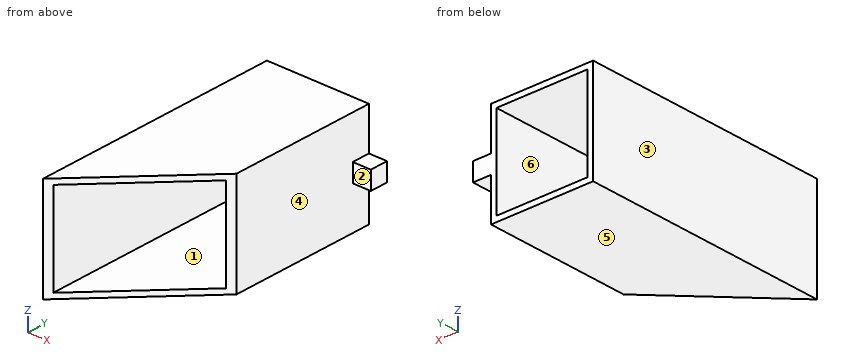
from build123d import *

# Parameters (mm, degrees)
CROQUIS1_W              = 56.5
CROQUIS1_H              = 56.5
SALIENTE_EXTRUIR1_DEPTH = 81.9
SALIENTE_EXTRUIR2_DEPTH = 56.5
VACIADO4_T              = -3
CROQUIS3_W              = 10
CROQUIS3_H              = 10
SALIENTE_EXTRUIR3_DEPTH = 10


with BuildPart() as part:
    # Croquis1 → Saliente-Extruir1 (new body)
    with BuildSketch(Plane(origin=(0, 0, 0), x_dir=(1, 0, 0), z_dir=(0, 1, 0))):
        with Locations((28.25, 28.25)):
            Rectangle(CROQUIS1_W, CROQUIS1_H)
    extrude(amount=SALIENTE_EXTRUIR1_DEPTH)

    # Croquis2 → Saliente-Extruir2 (add)
    with BuildSketch(Plane.XY):
        Polygon((0, 0), (0, -56.5), (56.5, 0), align=None)
    extrude(amount=-SALIENTE_EXTRUIR2_DEPTH)

    # Vaciado4
    vaciado4_openings = [part.faces().sort_by_distance(p)[0] for p in [
        (28.25, 81.9, -28.25),
        (28.25, -28.25, -28.25),
    ]]
    offset(amount=VACIADO4_T, openings=vaciado4_openings, kind=Kind.INTERSECTION)

    # Croquis3 → Saliente-Extruir3 (add)
    with BuildSketch(Plane(origin=(0, 81.9, 0), x_dir=(1, 0, 0), z_dir=(0, 1, 0))):
        with Locations((61.5, 28.25)):
            Rectangle(CROQUIS3_W, CROQUIS3_H)
    extrude(amount=-SALIENTE_EXTRUIR3_DEPTH)


solid = part.part
Build history of the part. All positions in model axes, mm. Face numbers are marked on the shaded views. A direction names the side the tool comes from. Give positions to 0.01 mm unless a question says otherwise; leave off trailing zeros. Loops run counter-clockwise (first coordinate to the right, second up) from the corner with the lowest first, then second, coordinate; pieces in that order, holes last. Notation, with made-up numbers: (-36.5, -29.75) -> (1.5, -29.75) arc R13 ccw to (1.5, -13.75) -> close; hole circle Ø6 at (-16.75, 17.25). An arc over 180 degrees is marked (long way). Answer in a Markdown table with one row per item.
Item 1: Slice it at A-A on z = -4.5. Write the cut outline in (x, y), plus the area to 3 significant figures.
Findings below:
| item | result |
|---|---|
| outline | (0, -56.5) -> (3, -53.5) -> (3, 81.9) -> (0, 81.9) -> close; (53.5, -3) -> (56.5, 0) -> (56.5, 81.9) -> (53.5, 81.9) -> close |
| area | 661 mm² |
Item 2: Probe line 1 along Z through (x, y) = (39, 0); line 2 along X through (y, z) = (37, -26.5); line 3 along X through (y, z) = (-19, -38). List the from-to ranges inside material, lowest first. Write a range as [from, to].
Findings below:
| item | result |
|---|---|
| line 1 | z = [-56.5, -53.5], [-3, 0] |
| line 2 | x = [0, 3], [53.5, 56.5] |
| line 3 | x = [0, 3] |
Item 3: Tool access for the marked faces 1, 2 and 3: list every direction of +Z, -Z, +X, -X, +Y, -Y with a clear straight run to the whole face (end or side of a thin tool).
Findings below:
| item | result |
|---|---|
| face 1 | +Y, -Y |
| face 2 | +Z, -Z, +X, -Y |
| face 3 | +Z, -Z, -X, +Y, -Y |
Item 4: Slice it at B-B on x = 9. Write the cut outline in (y, z), plus the area to 3 significant figures.
Findings below:
| item | result |
|---|---|
| outline | (-47.5, -56.5) -> (81.9, -56.5) -> (81.9, -53.5) -> (-47.5, -53.5) -> close; (-47.5, -3) -> (81.9, -3) -> (81.9, 0) -> (-47.5, 0) -> close |
| area | 776 mm² |
Item 5: Mould opens along Z. For the marked faces 4, 5 and 6 say: pulls with the +Z half, pulls with the -Z half, needs draft (parallel to the pull), parting line crosses it, or undercut.
Findings below:
| item | result |
|---|---|
| face 4 | needs draft |
| face 5 | pulls with the -Z half |
| face 6 | undercut |
Item 6: Slice it at C-C on y = 66.5. Write the cut outline in (x, z), plus the area to 3 significant figures.
Findings below:
| item | result |
|---|---|
| outline | (0, -56.5) -> (56.5, -56.5) -> (56.5, 0) -> (0, 0) -> close; hole (3, -53.5) -> (53.5, -53.5) -> (53.5, -3) -> (3, -3) -> close |
| area | 642 mm² |
Item 7: Slice it at D-D on y = -7. Write the cut outline in (x, z).
Findings below:
| item | result |
|---|---|
| outline | (0, -56.5) -> (49.5, -56.5) -> (49.5, -53.5) -> (3, -53.5) -> (3, -3) -> (49.5, -3) -> (49.5, 0) -> (0, 0) -> close |
Item 8: Flat gauge pin, fed straight in: P1, Ø11, axis at x = 63, y = 74.5, coming from the +Z side. Where does the tip first touch, or does it go through?
Findings below:
| item | result |
|---|---|
| P1 | stops at z = -23.25 |
